For this review, take the finished solid that the model builds, in its own axes (mm). Face numbers are marked on the shaded views. A direction names the side the tool comes from. Give positions to 0.01 mm unless a question says otherwise; leave off trailing zeros. Order: outer loops, then holes, each group sorted by start corner. A loop starts at its lowest first (then second) coordinate and runs counter-clockwise, first axis right, second up.
Item 1: For P1, Ø10.5, axis at x = 3, y = 1.5, coming from the +Z side; P2, Ø3.5, axis at x = 5, z = 3, coming from the -Y side; P3, Ø2.5, axis at x = 3.5, z = 3, coming from the +Y side, all flat-tipped, find the tip position at first contact; note any pin that passes through.
Item 2: Consider section A-A (x = -4.5). Give the boundary of the cut face in (y, z).
Item 3: Consider section D-D (z = 78.5). Give the boundary of the cut face in (x, y).
Item 4: Consider section C-C (y = 5). Give the boundary of the cut face in (x, z).
Item 5: Consider section B-B (z = 20.5). Give the boundary of the cut face in (x, y), plus the area to 3 significant figures.
Item 6: For probe 1 along Y at (x, z) = (-3, 11); probe 2 along Z at (x, y) = (34.5, -9); probe 3 along Y at (x, z) = (13.5, 23), list the stretches that pass through material, from the lowest coordinate up.
Item 7: The part is to be moulded in two halves that separate along Y. For the marked faces 1, 2 and 3, say which applies: released by +Y, released by -Y, zero draft, split by the parting line, or undercut.
Item 8: Machinability: for the marked faces 4 and 5, which of the approach directions +Z, -Z, +X, -X, +Y, -Y give a long, thin tool a straight path to every point of the face, cutting with its end or side? Answer none if there is none.
```python
from build123d import *

# Parameters (mm, degrees)
F1_DEPTH = 5
F2_DEPTH = 100
F3_DEPTH = 2
F5_DEPTH = 96


with BuildPart() as f1:
    # F0 (on Top) → F1 (new body)
    with BuildSketch(Plane.XY):
        Polygon((49.977495, 44.5), (0, 43), (-50, 43), (-50, -43), (0, -43), (49.977495, -44.5), (54.977495, -44.5), (54.977495, 44.650068), align=None)
        Polygon((0, -8), (0, 8), (9.5, 8), (9.5, 0), (9.5, -8), align=None, mode=Mode.SUBTRACT)
    extrude(amount=F1_DEPTH)

    # F0 (on Top) → F2 (join)
    with BuildSketch(Plane.XY):
        Polygon((-50, 43), (0, 43), (49.977495, 44.5), (54.977495, 44.650068), (54.977495, 49.652319), (-0.075017, 48), (-55, 48), (-55, -48), (-0.075017, -48), (54.977495, -49.652319), (54.977495, -44.5), (49.977495, -44.5), (0, -43), (-50, -43), align=None)
    extrude(amount=F2_DEPTH)

    # F0 (on Top) → F3 (join)
    with BuildSketch(Plane.XY):
        Polygon((9.5, 8), (0, 8), (0, -8), (9.5, -8), (9.5, 0), align=None)
    extrude(amount=F3_DEPTH)

    # F4 (on face) → F5 (cut)
    with BuildSketch(Plane.XZ.offset(48)):
        Polygon((-55, 0), (-48.205912, 0), (-14.9364, 100), (-55, 100), align=None)
    extrude(amount=-F5_DEPTH, mode=Mode.SUBTRACT)


solid = f1.part
```
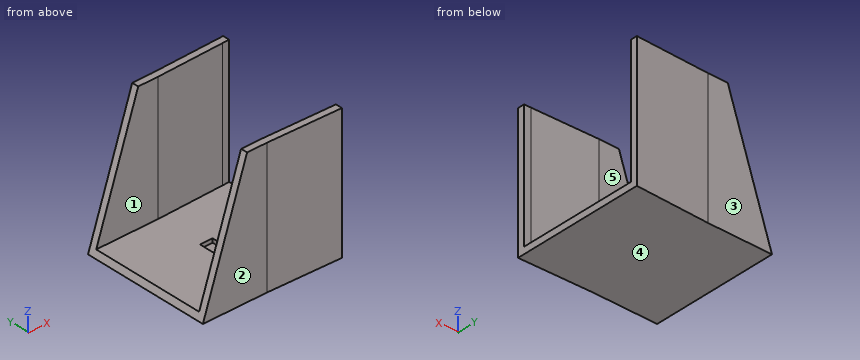
Resolved:
1. P1: stops at z = 5
1. P2: stops at y = -48.2
1. P3: stops at y = 48.14
2. outline: (-48, 0) - (48, 0) - (48, 100) - (43, 100) - (43, 5) - (-43, 5) - (-43, 100) - (-48, 100) - close
3. outline: (-22.09, -48) - (-0.08, -48) - (54.98, -49.65) - (54.98, -44.5) - (49.98, -44.5) - (0, -43) - (-22.09, -43) - close; (-22.09, 43) - (0, 43) - (54.98, 44.65) - (54.98, 49.65) - (-0.08, 48) - (-22.09, 48) - close
4. outline: (-48.21, 0) - (54.98, 0) - (54.98, 5) - (9.5, 5) - (9.5, 2) - (0, 2) - (0, 5) - (-46.54, 5) - close
5. outline: (-41.39, -48) - (-0.08, -48) - (54.98, -49.65) - (54.98, -44.5) - (49.98, -44.5) - (0, -43) - (-41.39, -43) - close; (-41.39, 43) - (0, 43) - (54.98, 44.65) - (54.98, 49.65) - (-0.08, 48) - (-41.39, 48) - close
5. area: 964 mm2
6. probe 1: y = -48 to -43, 43 to 48
6. probe 2: z = 0 to 5
6. probe 3: y = -48.41 to -43.41, 43.41 to 48.41
7. face 1: undercut
7. face 2: released by -Y
7. face 3: released by +Y
8. face 4: -Z, +X, -X, +Y, -Y
8. face 5: +Z, +X, -X
